Can you work these out from the model? Positions are in its coordinate system, mm. Face numbers are marked on the shaded views. A direction names the side the tool comes from. Round coordinates to 2 decimals unless told otherwise and drop trailing zeros. Write each loop counter-clockwise with the first axis right and the second up, starting at its lowest first coordinate (ties: lowest second). Pieces come first, ordered by that corner, then holes. Notation, with made-up numbers: (3, 21.5) -> (35, 21.5) arc R19 cw to (35, 48.5) -> close; hole circle Ø8 at (41, 17.25). An arc over 180 degrees is marked (long way). Write item = value, one per line. Start each with the question number.
1) If I drill on line 1 (Y direction, x = 4, z = -1.5); line 2 (Y direction, x = 2.5, z = -4.5); line 3 (X direction, y = -5.25, z = 2), over which ranges is the centre line in solid material (lowest first)?
2) I'm going to push flat-ended pins straight in: pin 1 (4 mm diameter, centred on x = 3.5, y = -8.5, fed in from -Z); pin 2 (1 mm diameter, centred on x = -3.5, z = -3, fed in from -Y); pin 3 (4 mm diameter, centred on x = 4, y = -10.5, fed in from -Z). Where does each tip first touch, or does it pass through?
3) For the marked faces 1 and 2, which set-ups out of +Z, -Z, +X, -X, +Y, -Y let a thin tool reach every point of the face, with its end or its side?
4) Imagine slicing it at A-A, the plane y = -1.5. Please give me the cut outline in (x, z), then the cut area to 3 significant figures.
5) Imagine slicing it at B-B, the plane y = -7.75. Please give me the cut outline in (x, z).
from build123d import *

# Parameters (mm, degrees)
BOSS_EXTRUDE1_DEPTH = 4
SKETCH4_R           = 2.5
BOSS_EXTRUDE2_DEPTH = 9


with BuildPart() as part:
    # Sketch1 → Boss-Extrude1 (new body)
    with BuildSketch(Plane(origin=(0, 0, 0), x_dir=(1, 0, 0), z_dir=(0, 1, 0))):
        Polygon((5.773502692, 0), (2.886751346, 5), (-2.886751346, 5), (-5.773502692, 0), (-2.886751346, -5), (2.886751346, -5), align=None)
    extrude(amount=-BOSS_EXTRUDE1_DEPTH)

    # Sketch3 → Cut-Revolve1 (revolve, cut)
    with BuildSketch(Plane.XY):
        Polygon((5.000002459, 0), (5.773502692, 0), (5.773502692, -0.446580568), align=None)
    revolve(axis=Axis((0, 1.337001122, 0), (0, -1, 0)), mode=Mode.SUBTRACT)

    # Sketch4 → Boss-Extrude2 (add)
    with BuildSketch(Plane.XZ.offset(4)):
        with Locations(Location((0, 0, 0), (0, 0, 90))):
            Circle(SKETCH4_R)
    extrude(amount=BOSS_EXTRUDE2_DEPTH)


solid = part.part
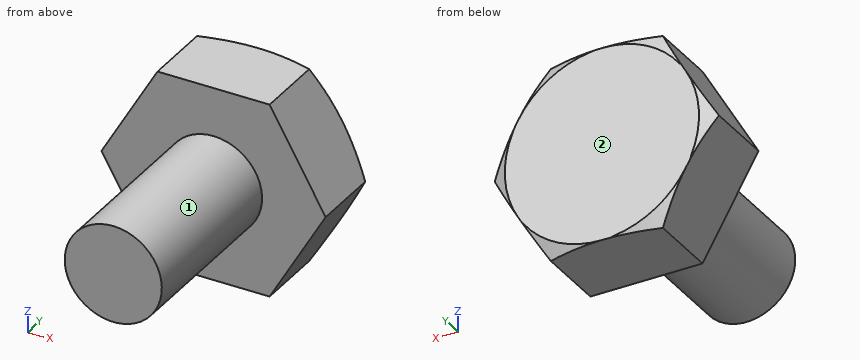
Reported:
q1.line_1 = -4 to 0
q1.line_2 = -4 to -0.09
q1.line_3 = -1.5 to 1.5
q2.pin_1 = -2
q2.pin_2 = -4
q2.pin_3 = -1.5
q3.face_1 = -Y
q3.face_2 = +Z, -Z, +X, -X, +Y
q4.outline = (-5.77, 0) -> (-2.89, -5) -> (2.89, -5) -> (5.77, 0) -> (2.89, 5) -> (-2.89, 5) -> close
q4.area = 86.6 mm²
q5.outline = circle Ø5 at (0, 0)
